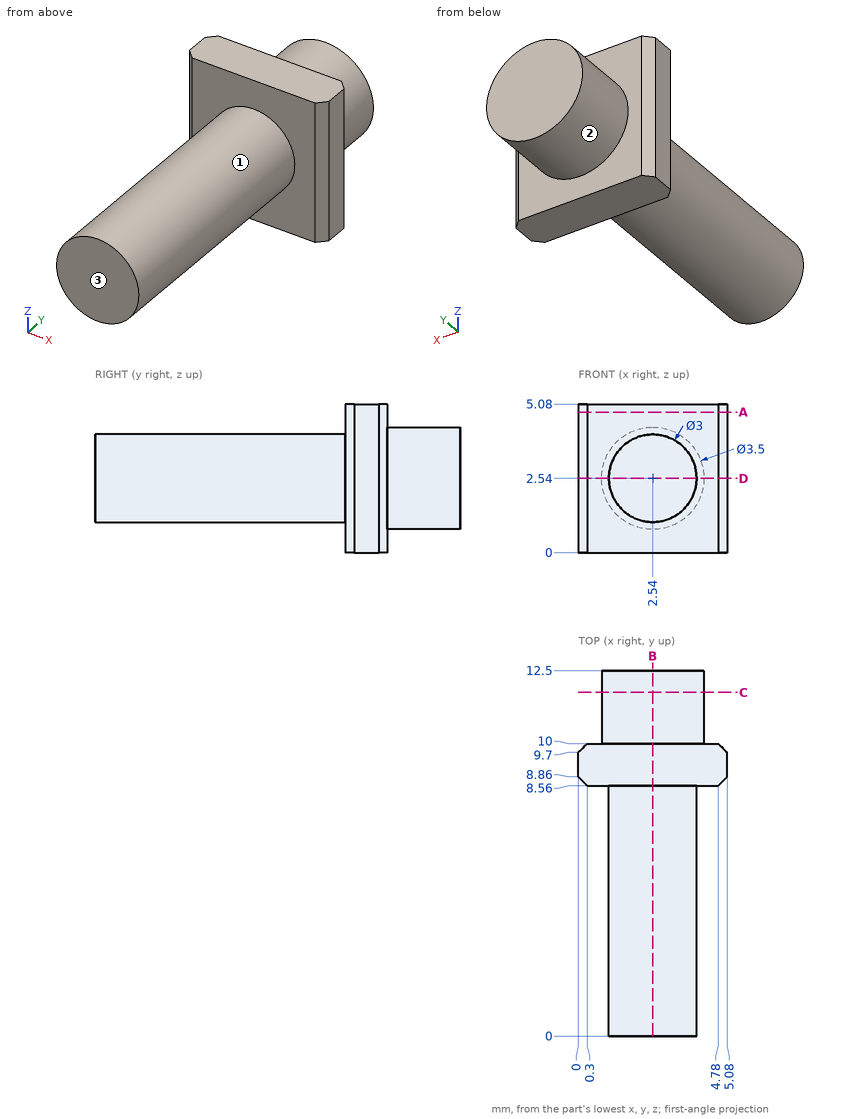
Input: dimensioned drawing with shaded views. Units: mm. Origin: part minimum x, y, z. A direction names the side the tool comes from. Give positions to 0.01 mm unless a question says otherwise; leave off trailing zeros. Loops run counter-clockwise (first coordinate to the right, second up) from the corner with the lowest first, then second, coordinate; pieces in that order, holes last. Notation, with made-up numbers: M -18.75,-5 L -3.75,-5 A20 ccw -3.75,28 Z; hole C -36,74 d6. An arc over 180 degrees is marked long. Put each result on its own line as item: value. Start each with the question number.
1) Cut plane A-A (z = 4.8). Output: boundary loops of the cut face in (x, y).
2) Cut plane D-D (z = 2.54). Output: boundary loops of the cut face in (x, y), then the cut area to 3 significant figures.
3) Access query for the marked faces 1, 2 and 3. Directions: +Z, -Z, +X, -X, +Y, -Y. A direction counts if a zero-diameter tool reaches every point of the face in a straight line with its end or side. Return the directions, or none.
4) Ray query, line 1 along Y through (x, z) = (0.5, 4.1); line 2 along Z through (x, y) = (1.6, 6.5); line 3 along Z through (x, y) = (1.5, 6.75). Return the intervals inside material, ascending.
5) Cut plane C-C (y = 11.75). Output: boundary loops of the cut face in (x, z).
6) Contact query for flat-ended pins moving along their axis: pin 1 (3 mm diameter, centred on x = 0.5, y = 3, fed in from +Z); pin 2 (1 mm diameter, centred on x = 1.5, z = 3.5, fed in from -Y). Output: stop coordinate, or through.
7) Cut plane B-B (x = 2.54). Output: boundary loops of the cut face in (y, z).
Verdict:
1. outline: M 0,8.86 L 0.3,8.56 L 4.78,8.56 L 5.08,8.86 L 5.08,9.7 L 4.78,10 L 0.3,10 L 0,9.7 Z
2. outline: M 0,8.86 L 0.3,8.56 L 1.04,8.56 L 1.04,0 L 4.04,0 L 4.04,8.56 L 4.78,8.56 L 5.08,8.86 L 5.08,9.7 L 4.78,10 L 4.29,10 L 4.29,12.5 L 0.79,12.5 L 0.79,10 L 0.3,10 L 0,9.7 Z
2. area: 41.6 mm2
3. face 1: -Y
3. face 2: +Y
3. face 3: +Z, -Z, +X, -X, -Y
4. line 1: 8.56 to 10
4. line 2: 1.37 to 3.71
4. line 3: 1.46 to 3.62
5. outline: C 2.54,2.54 d3.5
6. pin 1: z = 3.94
6. pin 2: y = 0
7. outline: M 0,1.04 L 8.56,1.04 L 8.56,0 L 10,0 L 10,0.79 L 12.5,0.79 L 12.5,4.29 L 10,4.29 L 10,5.08 L 8.56,5.08 L 8.56,4.04 L 0,4.04 Z
